Geometry check sheet. Reference: the model listing, model coordinates, mm. Face numbers are marked on the shaded views. A direction names the side the tool comes from. Give positions to 0.01 mm unless a question says otherwise; leave off trailing zeros. Order: outer loops, then holes, each group sorted by start corner. A loop starts at its lowest first (then second) coordinate and runs counter-clockwise, first axis right, second up. Notation, with made-up numbers: M -13,83.5 L -5,83.5 A16 cw -5,91.5 Z; hole C 54,7.25 d4. An arc over 180 degrees is marked long. Answer as a JSON object with one key per item and string values. Group by question number.
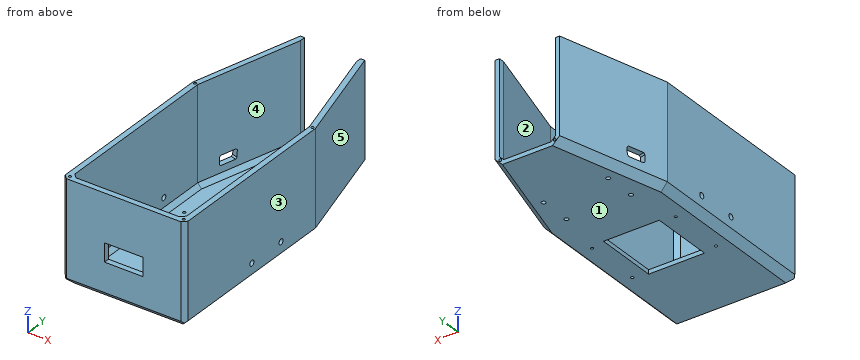
Autodesk Inventor part; units mm, degrees
ref_plane "YZ Plane" through (0, 0, 0) normal (1, 0, 0) x (0, 1, 0)
ref_plane "XZ Plane" through (0, 0, 0) normal (0, 1, 0) x (-1, 0, 0)
ref_plane "XY Plane" through (0, 0, 0) normal (0, 0, 1) x (1, 0, 0)
sketch "Sketch1" plane through (0, 0, 0) normal (0, 0, 1) x (1, 0, 0)
  line L0 (0, 0) -> (80, 0)
  line L1 (80, 0) -> (80, 125.359)
  line L2 (60, 200) -> (80, 125.359)
  line L3 (60, 200) -> (137.2741, 200) construction
  line L4 (0, 0) -> (0, 125.359)
  line L5 (20, 200) -> (0, 125.359)
  line L6 (84, 125.8856) -> (84, -4)
  line L7 (84, -4) -> (-4, -4)
  line L8 (-4, -4) -> (-4, 125.8856)
  line L9 (-4, 125.8856) -> (16.9307, 204)
  line L10 (63.0693, 204) -> (84, 125.8856)
  line L11 (20, 204) -> (20, 200)
  line L12 (60, 200) -> (60, 204)
  line L13 (16.9307, 204) -> (20, 204)
  line L14 (60, 204) -> (63.0693, 204)
  point P0 (40, 0)
  dimension "d0" = 80
  dimension "d4" = 75
  dimension "d5" = 4
extrude "Extrusion1" add sketch "Sketch1" along normal blind 70
sketch "Sketch2" plane through (0, 0, 0) normal (0, 0, -1) x (-1, 0, 0)
  line L0 (-16.9307, 204) -> (4, 125.8856)
  line L1 (-84, 125.8856) -> (-63.0693, 204)
  line L2 (-16.9307, 204) -> (-63.0693, 204)
  line L3 (-80, 125.359) -> (-80, 0)
  line L4 (-60, 200) -> (-80, 125.359)
  line L5 (-60, 204) -> (-60, 200)
  line L6 (-63.0693, 204) -> (-60, 204)
  line L7 (-84, 125.8856) -> (-63.0693, 204)
  line L8 (-84, -4) -> (-84, 125.8856)
  line L9 (4, -4) -> (-84, -4)
  line L10 (4, 125.8856) -> (4, -4)
  line L11 (-16.9307, 204) -> (4, 125.8856)
  line L12 (-20, 204) -> (-16.9307, 204)
  line L13 (-20, 200) -> (-20, 204)
  line L14 (0, 125.359) -> (-20, 200)
  line L15 (0, 0) -> (0, 125.359)
  line L16 (-80, 0) -> (0, 0)
extrude "Extrusion2" add sketch "Sketch2" along normal blind 3
chamfer "Chamfer1" distance 5 angle 45 5 edges at (40, -4, -3) (84, 60.9428, -3) (-4, 60.9428, -3) (6.4653, 164.9428, -3) (73.5347, 164.9428, -3)
chamfer "Chamfer2" distance 3 angle 45 7 edges at (20, 202, 0) (10, 162.6795, 0) (60, 202, 0) (70, 162.6795, 0) (80, 62.6795, 0) (0, 62.6795, 0) (40, 0, 0)
chamfer "Chamfer3" distance 3 angle 45 4 edges at (84, -4, 36) (-4, -4, 36) (0, 0, 36.5) (80, 0, 36.5)
sketch "Sketch3" plane through (0, 0, 70) normal (0, 0, 1) x (1, 0, 0)
  line L0 (77, 0) -> (78.5, 1.5)
  line L1 (81, -4) -> (82.5, -2.5)
  line L2 (78.5, 1.5) -> (82.5, -2.5)
  line L3 (79, 1) -> (82.5, -2.5)
  circle A0 centre (80.75, -0.75) radius 1
  line L4 (-4, -1) -> (-2.5, -2.5)
  line L5 (-2.5, -2.5) -> (1.5, 1.5)
  line L6 (0, 3) -> (3, 0)
  line L7 (1, 1) -> (-2.5, -2.5)
  circle A1 centre (-0.75, -0.75) radius 1
  line L8 (3, 124.964) -> (0, 125.359)
  line L9 (16.9307, 204) -> (-4, 125.8856)
  line L10 (80, 125.359) -> (77, 124.964)
  line L11 (84, -1) -> (84, 125.8856)
  line L12 (1, 125.2273) -> (-4, 125.8856)
  circle A2 centre (82, 125.6223) radius 1
  circle A3 centre (-2, 125.6223) radius 1
  point P0 (0, 0)
  dimension "d19" = 2
  dimension "d20" = 2
  dimension "d22" = 2
  dimension "d23" = 2
extrude "Extrusion3" cut sketch "Sketch3" against normal blind 5
sketch "Sketch4" plane through (22.1071, 204, -3) normal (0, 1, 0) x (1, 0, 0)
  line L0 (35.7859, 0) -> (40.9622, -5)
  line L1 (38.374, -2.5) -> (36.3929, -4.5)
  line L2 (34.8929, -3) -> (37.8929, -6)
  circle A0 centre (37.3835, -3.5) radius 1
  line L3 (-21.1071, 0) -> (56.8929, 0)
  line L4 (17.8929, 0) -> (17.8929, -26)
  circle A1 centre (-1.5976, -3.5) radius 1
  point P0 (-22.1071, -3)
  dimension "d26" = 2
extrude "Extrusion4" cut sketch "Sketch4" against normal blind 15
sketch "Sketch5" plane through (0, 0, 0) normal (0, 0, 1) x (1, 0, 0)
  line L0 (77, 3) -> (3, 3)
  line L1 (40, 3) -> (40, 43)
  line L2 (40, 43) -> (40, 113)
  line L3 (40, 78) -> (20, 78)
  line L4 (20, 78) -> (20, 55.5)
  line L5 (20, 55.5) -> (60, 55.5)
  line L6 (60, 55.5) -> (60, 100.5)
  line L7 (60, 100.5) -> (20, 100.5)
  line L8 (20, 100.5) -> (20, 78)
  line L9 (40, 78) -> (70, 78)
  line L10 (70, 78) -> (70, 98)
  circle A0 centre (70, 98) radius 1
  line L11 (70, 78) -> (70, 58)
  circle A1 centre (70, 58) radius 1
  circle A2 centre (10, 98) radius 1
  circle A3 centre (10, 58) radius 1
  line L12 (40, 113) -> (40, 133)
  line L13 (40, 133) -> (63.1521, 133)
  line L14 (63.1521, 133) -> (63.1521, 155.7076)
  circle A4 centre (63.1521, 155.7076) radius 1.5
  circle A5 centre (63.1521, 133) radius 1.5
  circle A6 centre (16.8479, 155.7076) radius 1.5
  circle A7 centre (16.8479, 133) radius 1.5
  point P0 (0, 0)
  dimension "d29" = 40
  dimension "d30" = 70
  dimension "d31" = 20
  dimension "d32" = 22.5
  dimension "d33" = 40
  dimension "d34" = 45
  dimension "d35" = 30
  dimension "d36" = 20
  dimension "d37" = 2
  dimension "d38" = 20
  dimension "d39" = 2
  dimension "d40" = 20
  dimension "d41" = 23.1521
  dimension "d42" = 22.7076
  dimension "d43" = 3
  dimension "d44" = 3
extrude "Extrusion5" cut sketch "Sketch5" against normal blind 40
sketch "Sketch7" plane through (-1, -4, 2) normal (0, -1, 0) x (1, 0, 0)
  line L0 (78, 68) -> (4, 68)
  line L1 (41, 68) -> (41, 34)
  line L2 (54.7, 34) -> (27.3, 34)
  line L3 (54.7, 34) -> (54.7, 20.8)
  line L4 (54.7, 20.8) -> (27.3, 20.8)
  line L5 (27.3, 34) -> (27.3, 20.8)
  point P0 (1, -2)
  dimension "d47" = 27.4
  dimension "d48" = 34
  dimension "d49" = 13.2
extrude "Extrusion6" cut sketch "Sketch7" against normal blind 27.4
sketch "Sketch8" plane through (-4, 125.8856, 2) normal (-0.9659, 0.2588, 0) x (0, 0, 1)
  line L0 (-2, 13.7678) -> (-2, 10.7678)
  line L1 (-2, 35.7017) -> (-2, 32.7017)
  line L2 (3.9828, 34.5121) -> (3.9828, 12.5782)
  line L3 (3.9828, 23.5451) -> (5.9828, 23.5451)
  line L4 (5.9828, 23.5451) -> (12.9828, 23.5451)
  line L5 (12.9828, 23.5451) -> (12.9828, 30.2951)
  line L6 (12.9828, 30.2951) -> (12.9828, 16.7951)
  line L7 (12.9828, 16.7951) -> (5.9828, 16.7951)
  line L8 (5.9828, 16.7951) -> (5.9828, 29.9848)
  line L9 (5.9828, 29.9848) -> (12.9828, 30.2951)
  point P0 (-2, -120.5609)
  point P1 (12.9828, 30.2951)
  dimension "d52" = 2
  dimension "d53" = 7
  dimension "d54" = 6.75
  dimension "d55" = 13.5
extrude "Extrusion7" cut sketch "Sketch8" against normal blind 9
chamfer "Chamfer4" distance 1 angle 45 4 edges at (5.7728, 154.6308, 14.9828) (2.2788, 141.5908, 14.9828) (2.2788, 141.5908, 7.9828) (5.6925, 154.331, 7.9828)
sketch "Sketch9" plane through (-4, 125.8856, 2) normal (-1, 0, 0) x (0, 0, 1)
  line L0 (1, -0.5266) -> (1, -122.8856)
  line L1 (1, -48.8247) -> (7.6436, -48.8247)
  line L2 (7.6436, -48.8247) -> (7.6436, -34.3247)
  line L3 (7.6436, -34.3247) -> (7.6436, -63.3247)
  circle A0 centre (7.6436, -34.3247) radius 2
  circle A1 centre (7.6436, -63.3247) radius 2
  point P0 (-2, -125.8856)
  dimension "d61" = 14.5
  dimension "d62" = 29
  dimension "d63" = 4
  dimension "d64" = 4
extrude "Extrusion8" cut sketch "Sketch9" against normal blind 999
equation "\"d45\" = d33"
equation "\"d50\" = d47"
properties part number "the box"
1. Cross-section at B-B (z = 25). Record the cut outline in (x, y).
2. Cross-section at A-A (y = 68). Record the cut outline in (x, z).
3. Release check for a two-part mould opening along X. For the marked faces 1, 2 and 3 record: released by +X, released by -X, zero draft, split by the parting line, or undercut.
4. Depth check by flat-ended pin: pin 1 (1.5 mm diameter, centred on y = 71.5, z = -1.5, fed in from -X); pin 2 (1.6 mm diameter, centred on x = -2, y = 125.5, fed in from +Z); pin 3 (5 mm diameter, centred on x = 18.5, y = 106, fed in from +Z). Enter the tip coordinate at first touch or a pass-through.
5. Cross-section at D-D (z = 39). Record the cut outline in (x, y), and give its area (3 significant figures).
6. Access from +Z, -Z, +X, -X, +Y, -Y to the whole of each face (thin tool, end or side, straight path). Record for the marked faces 4 and 5.
7. Cross-section at C-C (x = 32). Record the cut outline in (y, z), and give its area (3 significant figures).
8. Thickness scan on line 1 along X through (y, z) = (-0.75, 68.6); line 2 along X through (y, z) = (81, 10.5); line 3 along Z through (x, y) = (26.5, 29). Record the ranges inside material, lowest first. Write a range as [from, to].
Report:
{
 "1": {"outline": "M -4,-1 L -1,-4 L 26.3,-4 L 26.3,0 L 3,0 L 0,3 L 0,125.36 L 20,200 L 20,204 L 16.93,204 L -4,125.89 Z; M 53.7,-4 L 81,-4 L 84,-1 L 84,125.89 L 63.07,204 L 60,204 L 60,200 L 80,125.36 L 80,3 L 77,0 L 53.7,0 Z"},
 "2": {"outline": "M -4,2 L 1,-3 L 20,-3 L 20,0 L 3,0 L 0,3 L 0,70 L -4,70 Z; M 60,-3 L 79,-3 L 84,2 L 84,70 L 80,70 L 80,3 L 77,0 L 60,0 Z"},
 "3": {"face 1": "zero draft", "face 2": "undercut", "face 3": "released by +X"},
 "4": {"pin 1": "stops at x = -1.25", "pin 2": "stops at z = 65", "pin 3": "stops at z = 0"},
 "5": {"outline": "M -4,-1 L -1,-4 L 81,-4 L 84,-1 L 84,125.89 L 63.07,204 L 60,204 L 60,200 L 80,125.36 L 80,3 L 77,0 L 3,0 L 0,3 L 0,125.36 L 20,200 L 20,204 L 16.93,204 L -4,125.89 Z", "area": "2,000 mm2"},
 "6": {"face 4": "+Z", "face 5": "+Z, -Z, +X, +Y"},
 "7": {"outline": "M -4,2 L 1,-3 L 55.5,-3 L 55.5,0 L 3,0 L 0,3 L 0,22.8 L -4,22.8 Z; M -4,36 L 0,36 L 0,70 L -4,70 Z; M 100.5,-3 L 204,-3 L 204,0 L 100.5,0 Z", "area": "708 mm2"},
 "8": {"line 1": "x = [-4, -1.75], [0.25, 79.75], [81.75, 84]", "line 2": "x = [-4, 0], [80, 84]", "line 3": "z = [-3, 0]"}
}
